Geometry: final body of the model. Coordinates: model frame, mm. A direction names the side the tool comes from. Round coordinates to 2 decimals unless told otherwise and drop trailing zeros. Loops run counter-clockwise (first coordinate to the right, second up) from the corner with the lowest first, then second, coordinate; pieces in that order, holes last. Notation, with made-up numbers: M 64.25,10.25 L 117.25,10.25 A25 cw 117.25,28.25 Z; hole C 82,-27.5 d10. An arc over 180 degrees is marked long. Answer as a JSON object with one key per item and string values.
```python
from build123d import *

# Parameters (mm, degrees)
F0_R     = 5
F1_DEPTH = 3
F2_R     = 3
F3_DEPTH = 35
F4_SIZE  = 0.25


with BuildPart() as f1:
    # F0 (on Front) → F1 (new body)
    with BuildSketch(Plane.XZ):
        Circle(F0_R)
    extrude(amount=F1_DEPTH)

    # F2 (on face) → F3 (join)
    with BuildSketch(Plane.XZ.offset(3)):
        Circle(F2_R)
    extrude(amount=F3_DEPTH)

    # F4
    f4_edges = [f1.edges().sort_by_distance(p)[0] for p in [
        (-5, 0, 0),
        (-5, -3, 0),
        (-3, -38, 0),
    ]]
    chamfer(f4_edges, length=F4_SIZE)


solid = f1.part
```
1) Cut plane B-B on x = 0. Return the cut outline in (y, z).
Geometry results:
{"outline": "M -38,-2.75 L -37.75,-3 L -3,-3 L -3,-4.75 L -2.75,-5 L -0.25,-5 L 0,-4.75 L 0,4.75 L -0.25,5 L -2.75,5 L -3,4.75 L -3,3 L -37.75,3 L -38,2.75 Z"}
2) Set-up query: faces 1 (the face through (0, -38, 0)), 2 (the face through (3, -3, -1)). Return all of +Z, -Z, +X, -X, +Y, -Y with unobstructed straight access to the full face (end or side cutting, diameter ignored); none if empty.
Geometry results:
{"face 1": "+Z, -Z, +X, -X, -Y", "face 2": "-Y"}
3) Cut plane A-A on z = 0. Return the cut outline in (x, y).
Geometry results:
{"outline": "M -5,-2.75 L -4.75,-3 L -3,-3 L -3,-37.75 L -2.75,-38 L 2.75,-38 L 3,-37.75 L 3,-3 L 4.75,-3 L 5,-2.75 L 5,-0.25 L 4.75,0 L -4.75,0 L -5,-0.25 Z"}
4) Line query: probe 1 along Y at (x, z) = (-3.5, -1.75); probe 2 along Z at (x, y) = (-0.25, -8.5); probe 3 along Y at (x, z) = (-2, -4.5). Output: solid intervals per line, ascending.
Geometry results:
{"probe 1": "-3 to 0", "probe 2": "-2.99 to 2.99", "probe 3": "-2.83 to -0.17"}
5) First-contact query: pin 1 (5 mm diameter, centred on x = -0.5, y = -11, fed in from +Z); pin 2 (3 mm diameter, centred on y = -30.5, z = 3, fed in from -X); pin 3 (6 mm diameter, centred on x = -2, y = -32.5, fed in from -Z). Flat tips, straight axial feed; report the tip coordinate or a pass-through.
Geometry results:
{"pin 1": "z = 3", "pin 2": "x = -2.6", "pin 3": "z = -3"}
6) Cut plane C-C on y = -33. Return the cut outline in (x, z).
Geometry results:
{"outline": "C 0,0 d6"}
